The figure shows three views and two pictorial views of one solid part (mm, origin at its lowest corner). Answer the questions. A direction names the side the tool comes from. Coordinates: 2 decimals unless noted, no trailing zeros. Order: outer loops, then holes, each group sorted by start corner. A loop starts at its lowest first (then second) coordinate and runs counter-clockwise, first axis right, second up. Notation, with made-up numbers: (72, -38) - (103, -38) arc R25 ccw to (103, -1) - close; hole circle Ø5 at (38, 27). An arc over 180 degrees is marked (long way). Use one line per item in the form item = value.
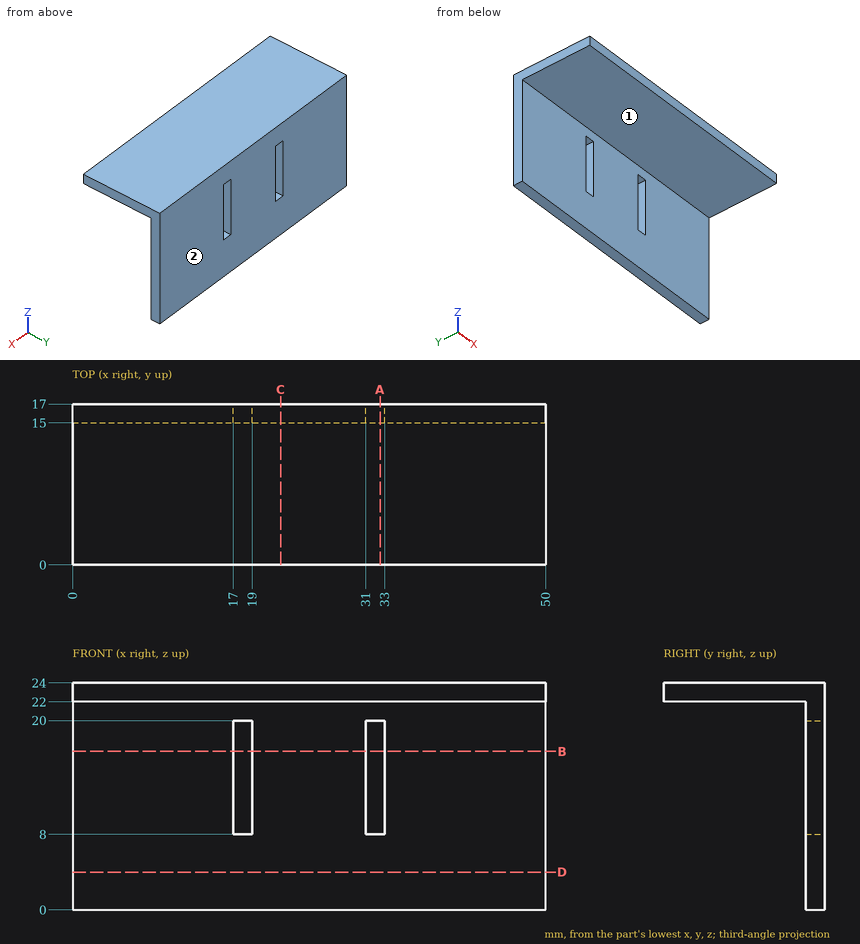
(1) Section D-D, the plane z = 4 is taken. Write down the section's boundary in (x, y), then the cut area to 3 significant figures.
Answer list:
outline = (0, 15) - (50, 15) - (50, 17) - (0, 17) - close
area = 100 mm2
(2) Straight lines are drawn through the part: L1, parallel to X at y = 16, z = 18; L2, parallel to Y at x = 34, z = 21.5; L3, parallel to Z at x = 15, y = 1. For each, find the intervals that lie inside material, in ascending order.
Answer list:
L1 = 0 to 17, 19 to 31, 33 to 50
L2 = 15 to 17
L3 = 22 to 24
(3) Section B-B, the plane z = 16.75 is taken. Write down the section's boundary in (x, y), then the cut area to 3 significant figures.
Answer list:
outline = (0, 15) - (17, 15) - (17, 17) - (0, 17) - close; (19, 15) - (31, 15) - (31, 17) - (19, 17) - close; (33, 15) - (50, 15) - (50, 17) - (33, 17) - close
area = 92.0 mm2
(4) Section A-A, the plane x = 32.5 is taken. Write down the section's boundary in (y, z).
Answer list:
outline = (0, 22) - (15, 22) - (15, 20) - (17, 20) - (17, 24) - (0, 24) - close; (15, 0) - (17, 0) - (17, 8) - (15, 8) - close
(5) Given pin 1 Ø1.6 at (x, y) = (32, 16) entering from -Z; pin 2 Ø10 at (x, y) = (5.5, 3.5) entering from -Z, each flat-ended and moving along its own axis, determine where each tip first touches the part or whether it passes through.
Answer list:
pin_1 = 0
pin_2 = 22
(6) Section C-C, the plane x = 22 is taken. Write down the section's boundary in (y, z).
Answer list:
outline = (0, 22) - (15, 22) - (15, 0) - (17, 0) - (17, 24) - (0, 24) - close
(7) Which of the six approach directions +Z, -Z, +X, -X, +Y, -Y give full straight-line access (tool end or side, diameter ignored) to the marked faces 1 and 2?
Answer list:
face_1 = -Z, +X, -X, -Y
face_2 = +Z, -Z, +X, -X, +Y
